Can you work these out from the model? Positions are in its coordinate system, mm. Face numbers are marked on the shaded views. A direction names the side the tool comes from. Round coordinates to 2 decimals unless told otherwise and drop trailing zeros. Write each loop counter-clockwise with the first axis right and the second up, starting at its lowest first coordinate (ties: lowest second). Pieces come first, ordered by that corner, then holes. Notation, with made-up numbers: (89.25, 73) -> (133.25, 73) arc R32 cw to (133.25, 102) -> close; hole circle Ø1 at (68.5, 47). An arc over 180 degrees is marked (long way). Use CSV: the item, a comma, the result in double quotes.
Autodesk Inventor part; units mm, degrees
ref_plane "YZ Plane" through (0, 0, 0) normal (1, 0, 0) x (0, 1, 0)
ref_plane "XZ Plane" through (0, 0, 0) normal (0, 1, 0) x (-1, 0, 0)
ref_plane "XY Plane" through (0, 0, 0) normal (0, 0, 1) x (1, 0, 0)
sketch "Skizze1" plane through (0, 0, 0) normal (0, 1, 0) x (-1, 0, 0)
  line L0 (0, 0) -> (0, -8.5)
  line L1 (0, -8.5) -> (8.5, -8.5)
  line L2 (8.5, -8.5) -> (8.5, -14.5)
  line L3 (8.5, -14.5) -> (0, -14.5)
  line L4 (0, -14.5) -> (0, -23)
  line L5 (0, -23) -> (-6, -23)
  line L6 (-6, -23) -> (-6, -14.5)
  line L7 (-6, -14.5) -> (-14.5, -14.5)
  line L8 (-14.5, -14.5) -> (-14.5, -8.5)
  line L9 (-14.5, -8.5) -> (-6, -8.5)
  line L10 (-6, 0) -> (0, 0)
  line L11 (-6, -8.5) -> (-6, 0)
  dimension "d0" = 23
  dimension "d1" = 23
  dimension "d2" = 6
  dimension "d3" = 6
  dimension "d4" = 8.5
  dimension "d5" = 8.5
  dimension "d6" = 8.5
extrude "Extrusion1" add sketch "Skizze1" along normal blind 4
sketch "Skizze2" plane through (0, 4, 0) normal (0, 1, 0) x (1, 0, 0)
  line L0 (3, 1.9793) -> (1.25, 5.0104)
  line L1 (1.25, 5.0104) -> (4.75, 5.0104)
  line L2 (4.75, 5.0104) -> (3, 1.9793)
  line L3 (6, 23) -> (0, 23)
  line L4 (0, 0) -> (6, 0)
  line L5 (3, 21.0207) -> (4.75, 17.9896)
  line L6 (4.75, 17.9896) -> (1.25, 17.9896)
  line L7 (1.25, 17.9896) -> (3, 21.0207)
  line L8 (-6.5207, 11.5) -> (-3.4896, 13.25)
  line L9 (-3.4896, 13.25) -> (-3.4896, 9.75)
  line L10 (-3.4896, 9.75) -> (-6.5207, 11.5)
  line L11 (12.5207, 11.5) -> (9.4896, 9.75)
  line L12 (9.4896, 9.75) -> (9.4896, 13.25)
  line L13 (9.4896, 13.25) -> (12.5207, 11.5)
  line L14 (-8.5, 14.5) -> (-8.5, 8.5)
  line L15 (14.5, 8.5) -> (14.5, 14.5)
  point P0 (3, 4)
  point P1 (3, 19)
  point P2 (-4.5, 11.5)
  point P3 (10.5, 11.5)
  dimension "d9" = 4
  dimension "d10" = 3
  dimension "d11" = 4
  dimension "d12" = 4
  dimension "d13" = 4
  dimension "d14" = 3
  dimension "d15" = 3
  dimension "d16" = 3
  dimension "d17" = 3.5
  dimension "d18" = 3.5
  dimension "d19" = 3.5
  dimension "d20" = 3.5
extrude "Extrusion2" cut sketch "Skizze2" against normal blind 0.5
fillet "Rundung1" radius 1 12 edges at (6, 4, -4.25) (3, 4, 0) (0, 4, -4.25) (10.25, 4, -8.5) (10.25, 4, -14.5) (14.5, 4, -11.5) (6, 4, -18.75) (3, 4, -23) (0, 4, -18.75) (-4.25, 4, -14.5) (-8.5, 4, -11.5) (-4.25, 4, -8.5)
sketch "Skizze3" plane through (0, 0, 0) normal (0, -1, 0) x (1, 0, 0)
  line L0 (15.5, -15.5) -> (7, -15.5)
  line L1 (7, -15.5) -> (7, -24)
  line L2 (7, -24) -> (-1, -24)
  line L3 (-1, -24) -> (-1, -15.5)
  line L4 (-1, -15.5) -> (-9.5, -15.5)
  line L5 (-9.5, -15.5) -> (-9.5, -7.5)
  line L6 (-9.5, -7.5) -> (-1, -7.5)
  line L7 (-1, -7.5) -> (-1, 1)
  line L8 (-1, 1) -> (7, 1)
  line L9 (7, 1) -> (7, -7.5)
  line L10 (14.5, -8.5) -> (6, -8.5)
  line L11 (7, -7.5) -> (15.5, -7.5)
  line L12 (15.5, -7.5) -> (15.5, -15.5)
  point P0 (0, 0)
  point P1 (14.5, -14.5)
  point P2 (6, -23)
  point P3 (-8.5, -8.5)
  point P4 (0, -8.5)
  point P5 (6, 0)
  dimension "d25" = 8.5
  dimension "d26" = 25
  dimension "d27" = 25
  dimension "d28" = 8
  dimension "d29" = 8
  dimension "d30" = 8
  dimension "d31" = 8
  dimension "d32" = 8.5
  dimension "d33" = 8.5
  dimension "d34" = 8.5
  dimension "d35" = 8.5
  dimension "d36" = 8.5
extrude "Extrusion3" add sketch "Skizze3" along normal blind 3
properties part number "Kreuz"
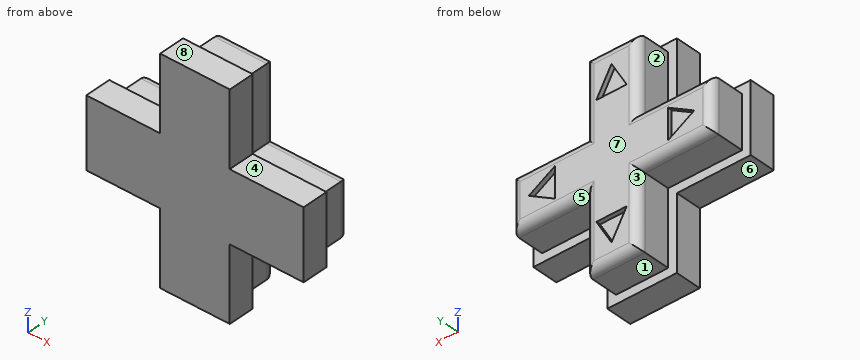
Q1. Suppose I cut it at A-A (y = 1.5). Write out the boundary of the cut face in (x, z).
Resolved:
outline,"(-8.5, -14.5) -> (0, -14.5) -> (0, -23) -> (6, -23) -> (6, -14.5) -> (14.5, -14.5) -> (14.5, -8.5) -> (6, -8.5) -> (6, 0) -> (0, 0) -> (0, -8.5) -> (-8.5, -8.5) -> close"
Q2. Suppose I cut it at B-B (x = 8). Write out the boundary of the cut face in (y, z), and give its area (3 significant figures).
Resolved:
outline,"(-3, -15.5) -> (0, -15.5) -> (0, -14.5) -> (3, -14.5) arc R1 ccw to (4, -13.5) -> (4, -9.5) arc R1 ccw to (3, -8.5) -> (0, -8.5) -> (0, -7.5) -> (-3, -7.5) -> close"
area,"47.6 mm^2"
Q3. Please list where these lines run through material, in increasing order: probe 1 along Z at (x, y) = (9.25, -1); probe 2 along X at (y, z) = (-1, -20.75); probe 3 along Z at (x, y) = (14, 1.25).
Resolved:
probe 1,"z = -15.5 to -7.5"
probe 2,"x = -1 to 7"
probe 3,"z = -14.5 to -8.5"
Q4. Suppose I cut it at D-D (y = -2). Write out the boundary of the cut face in (x, z), and give its area (3 significant figures).
Resolved:
outline,"(-9.5, -15.5) -> (-1, -15.5) -> (-1, -24) -> (7, -24) -> (7, -15.5) -> (15.5, -15.5) -> (15.5, -7.5) -> (7, -7.5) -> (7, 1) -> (-1, 1) -> (-1, -7.5) -> (-9.5, -7.5) -> close"
area,"336 mm^2"
Q5. Will these pins go through, and if not, where does the flat tip stop? P1, Ø2.5, axis at x = 11, y = -2, coming from the -Z side; P2, Ø1, axis at y = 1, z = -21, coming from the -X side; P3, Ø0.9, axis at x = -3, y = 1, coming from the +Z side.
Resolved:
P1,"stops at z = -15.5"
P2,"stops at x = 0"
P3,"stops at z = -8.5"
Q6. If we mould it in two halves opening along Z, with no side actions, what happens to the marked faces 6, 7 and 8? For each: released by +Z, released by -Z, zero draft, split by the parting line, or undercut.
Resolved:
face 6,"released by -Z"
face 7,"zero draft"
face 8,"released by +Z"
Q7. Suppose I cut it at C-C (z = -21.5). Write out the boundary of the cut face in (x, y).
Resolved:
outline,"(-1, -3) -> (7, -3) -> (7, 0) -> (6, 0) -> (6, 3) arc R1 ccw to (5, 4) -> (1, 4) arc R1 ccw to (0, 3) -> (0, 0) -> (-1, 0) -> close"
Q8. On a 3-axis mill with a long thin cutter (end or side, diameter ignored), from which of +Z, -Z, +X, -X, +Y, -Y can I reach the whole of each face in a straight line? I mean the marked faces 1, 2, 3, 4 and 5. Say none if no direction works.
Resolved:
face 1,"-Z, +X, -X, +Y"
face 2,"+Z, -X, +Y"
face 3,"-Z, -X, +Y"
face 4,"+Z, +X, +Y, -Y"
face 5,"-Z, +X, +Y"
